Check sheet for the modelled part. Datum: model origin and axes. Units: mm. Face numbers are marked on the shaded views. A direction names the side the tool comes from. Give positions to 0.01 mm unless a question says otherwise; leave off trailing zeros. Write each loop counter-clockwise with the first axis right and the second up, starting at its lowest first coordinate (ties: lowest second). Pieces come first, ordered by that corner, then holes. Notation, with made-up numbers: (8.25, -1) -> (44.25, -1) arc R6 ccw to (44.25, 10) -> close; hole circle Ø10 at (27, 5.5). An arc over 180 degrees is marked (long way). Answer as a JSON object with one key per item and string values.
from build123d import *

# Parameters (mm, degrees)
SKETCH1_W           = 25
SKETCH1_H           = 50
SKETCH1_R           = 3.4
BOSS_EXTRUDE1_DEPTH = 3
SKETCH2_W           = 50
SKETCH2_H           = 3
BOSS_EXTRUDE2_DEPTH = 8
SKETCH3_W           = 8
SKETCH3_H           = 50
BOSS_EXTRUDE3_DEPTH = 42
SKETCH4_R           = 2.65
CUT_EXTRUDE1_DEPTH  = 0.5
SKETCH5_R           = 5.802370205
CUT_EXTRUDE2_DEPTH  = 9
FILLET2_R           = 1
SKETCH6_R           = 12.6
BOSS_EXTRUDE4_DEPTH = 2
FILLET4_R           = 1
SKETCH8_R           = 1.589780168
SKETCH8_R_2         = 1.777428262
CUT_EXTRUDE3_DEPTH  = 10
SKETCH9_W           = 49.021678163
SKETCH9_H           = 20.976854622
CUT_EXTRUDE4_DEPTH  = 68.79439129
SKETCH11_R          = 2.1
CUT_EXTRUDE5_DEPTH  = 59.480168703
SKETCH14_R          = 2.6
CUT_EXTRUDE6_DEPTH  = 0.5
CUT_EXTRUDE7_DEPTH  = 10


with BuildPart() as part:
    # Sketch1 → Boss-Extrude1 (new body)
    with BuildSketch(Plane(origin=(0, 0, 0), x_dir=(1, 0, 0), z_dir=(0, 1, 0))):
        with Locations((2.276951673, 11.384758364)):
            Rectangle(SKETCH1_W, SKETCH1_H)
        with Locations(Location((1.276951673, 11.384758364, 0), (0, 0, 270))):
            Circle(SKETCH1_R, mode=Mode.SUBTRACT)
    extrude(amount=BOSS_EXTRUDE1_DEPTH)

    # Sketch2 → Boss-Extrude2 (add)
    with BuildSketch(Plane.ZY.offset(10.223048327)):
        with Locations((-11.384758364, 1.5)):
            Rectangle(SKETCH2_W, SKETCH2_H)
    extrude(amount=BOSS_EXTRUDE2_DEPTH)

    # Sketch3 → Boss-Extrude3 (add)
    with BuildSketch(Plane.XZ):
        with Locations((-14.223048327, -11.384758364)):
            Rectangle(SKETCH3_W, SKETCH3_H)
    extrude(amount=BOSS_EXTRUDE3_DEPTH)

    # Sketch4 → Cut-Extrude1 (cut)
    with BuildSketch(Plane(origin=(0, 3, 0), x_dir=(1, 0, 0), z_dir=(0, 1, 0))):
        with Locations(Location((-14.223048327, 32.384758364, 0), (0, 0, 270))):
            Circle(SKETCH4_R)
        with Locations(Location((-14.223048327, -9.615241636, 0), (0, 0, 270))):
            Circle(SKETCH4_R)
    cut_extrude1 = extrude(amount=-CUT_EXTRUDE1_DEPTH, mode=Mode.SUBTRACT)

    # Mirror1: Cut-Extrude1 across plane
    add(cut_extrude1.mirror(Plane.ZX.offset(-19.5)), mode=Mode.SUBTRACT)

    # Sketch5 → Cut-Extrude2 (cut)
    with BuildSketch(Plane.ZY.offset(18.223048327)):
        with Locations((-11.836279124, -21)):
            Circle(SKETCH5_R)
    extrude(amount=-CUT_EXTRUDE2_DEPTH, mode=Mode.SUBTRACT)

    # Fillet2
    fillet2_edges = [part.edges().sort_by_distance(p)[0] for p in [
        (-10.223048327, -21, -17.638649329),
    ]]
    fillet(fillet2_edges, radius=FILLET2_R)

    # Mirror2: Cut-Extrude1 across plane
    add(cut_extrude1.mirror(Plane.ZY.offset(1.723048327)), mode=Mode.SUBTRACT)

    # Sketch6 → Boss-Extrude4 (add)
    with BuildSketch(Plane(origin=(0, 3, 0), x_dir=(1, 0, 0), z_dir=(0, 1, 0))):
        with BuildLine():
            Line((14.776951673, 5.825082115), (14.776951673, 16.944434614))
            ThreePointArc((14.776951673, 16.944434614), (-13.323048327, 11.384758364), (14.776951673, 5.825082115))
        make_face()
        with Locations(Location((1.276951673, 11.384758364, 0), (0, 0, 270))):
            Circle(SKETCH6_R, mode=Mode.SUBTRACT)
    extrude(amount=BOSS_EXTRUDE4_DEPTH)

    # Fillet4
    # the kernel refuses this fillet: 1 mm, written as the material it takes off along each edge
    with BuildSketch(Plane(origin=(14.776951673, 5, -3.325082115), x_dir=(0, -1, 0), z_dir=(0, 0, -1))) as fillet4_piece_1:
        with BuildLine():
            CenterArc((FILLET4_R, FILLET4_R), FILLET4_R, 180, 90)
            Line((0, FILLET4_R), (0, 0))
            Line((0, 0), (FILLET4_R, 0))
        make_face()
    extrude(amount=16.119352499, mode=Mode.SUBTRACT)

    # Sketch8 → Cut-Extrude3 (cut)
    with BuildSketch(Plane(origin=(0, 3, 0), x_dir=(1, 0, 0), z_dir=(0, 1, 0))):
        with Locations(Location((1.276951673, 19.884758364, 0), (0, 0, 270))):
            Circle(SKETCH8_R)
        with Locations(Location((1.276951673, 2.884758364, 0), (0, 0, 270))):
            Circle(SKETCH8_R_2)
    extrude(amount=-CUT_EXTRUDE3_DEPTH, mode=Mode.SUBTRACT)

    # Sketch9 → Cut-Extrude4 (cut, through all)
    with BuildSketch(Plane.XY.offset(13.615241636)):
        with Locations((-9.733887409, 10.488427311)):
            Rectangle(SKETCH9_W, SKETCH9_H)
    extrude(amount=-CUT_EXTRUDE4_DEPTH, mode=Mode.SUBTRACT)

    # Sketch11 → Cut-Extrude5 (cut, through all)
    with BuildSketch(Plane(origin=(0, 0, 0), x_dir=(1, 0, 0), z_dir=(0, 1, 0))):
        with Locations(Location((-14.223048327, 32.384758364, 0), (0, 0, 270))):
            Circle(SKETCH11_R)
    cut_extrude5 = extrude(amount=-CUT_EXTRUDE5_DEPTH, mode=Mode.SUBTRACT)

    # Mirror3: Cut-Extrude5 across plane
    add(cut_extrude5.mirror(Plane.XY.offset(-11.384758364)), mode=Mode.SUBTRACT)

    # Sketch14 → Cut-Extrude6 (cut)
    with BuildSketch(Plane(origin=(0, 0, 0), x_dir=(1, 0, 0), z_dir=(0, 1, 0))):
        with Locations(Location((-14.223048327, -9.615241636, 0), (0, 0, 270))):
            Circle(SKETCH14_R)
    cut_extrude6 = extrude(amount=-CUT_EXTRUDE6_DEPTH, mode=Mode.SUBTRACT)

    # Mirror4: Cut-Extrude6 across plane
    add(cut_extrude6.mirror(Plane.XY.offset(-11.384758364)), mode=Mode.SUBTRACT)

    # Sketch15 → Cut-Extrude7 (cut)
    with BuildSketch(Plane(origin=(-10.223048327, 0, 0), x_dir=(0, 0, -1), z_dir=(1, 0, 0))):
        with BuildLine():
            ThreePointArc((-4.015241636, -4), (-6.136561979, -4.878679656), (-7.015241636, -7))
            Line((-7.015241636, -7), (-7.015241636, -16.15570602))
            ThreePointArc((-7.015241636, -16.15570602), (-6.136561979, -18.277026364), (-4.015241636, -19.15570602))
            Line((-4.015241636, -19.15570602), (3.027273521, -19.15570602))
            ThreePointArc((3.027273521, -19.15570602), (5.435051506, -14.673525074), (9.888641359, -12.213265275))
            Line((9.888641359, -12.213265275), (9.888641359, -7))
            ThreePointArc((9.888641359, -7), (9.009961702, -4.878679656), (6.888641359, -4))
            Line((6.888641359, -4), (-4.015241636, -4))
        make_face()
        with BuildLine():
            Line((13.783916889, -7), (13.783916889, -12.213265275))
            ThreePointArc((13.783916889, -12.213265275), (18.237506742, -14.673525074), (20.645284727, -19.15570602))
            Line((20.645284727, -19.15570602), (27.687799884, -19.15570602))
            ThreePointArc((27.687799884, -19.15570602), (29.809120227, -18.277026364), (30.687799884, -16.15570602))
            Line((30.687799884, -16.15570602), (30.687799884, -7))
            ThreePointArc((30.687799884, -7), (29.809120227, -4.878679656), (27.687799884, -4))
            Line((27.687799884, -4), (16.783916889, -4))
            ThreePointArc((16.783916889, -4), (14.662596546, -4.878679656), (13.783916889, -7))
        make_face()
        with BuildLine():
            ThreePointArc((20.645284727, -22.84429398), (18.237506742, -27.326474926), (13.783916889, -29.786734725))
            Line((13.783916889, -29.786734725), (13.783916889, -38))
            Line((13.783916889, -38), (27.687799884, -38))
            ThreePointArc((27.687799884, -38), (29.809120227, -37.121320344), (30.687799884, -35))
            Line((30.687799884, -35), (30.687799884, -25.84429398))
            ThreePointArc((30.687799884, -25.84429398), (29.809120227, -23.722973636), (27.687799884, -22.84429398))
            Line((27.687799884, -22.84429398), (20.645284727, -22.84429398))
        make_face()
        with BuildLine():
            ThreePointArc((9.888641359, -29.786734725), (5.435051506, -27.326474926), (3.027273521, -22.84429398))
            Line((3.027273521, -22.84429398), (-4.015241636, -22.84429398))
            ThreePointArc((-4.015241636, -22.84429398), (-6.136561979, -23.722973636), (-7.015241636, -25.84429398))
            Line((-7.015241636, -25.84429398), (-7.015241636, -35))
            ThreePointArc((-7.015241636, -35), (-6.136561979, -37.121320344), (-4.015241636, -38))
            Line((-4.015241636, -38), (9.888641359, -38))
            Line((9.888641359, -38), (9.888641359, -29.786734725))
        make_face()
    extrude(amount=-CUT_EXTRUDE7_DEPTH, mode=Mode.SUBTRACT)


solid = part.part
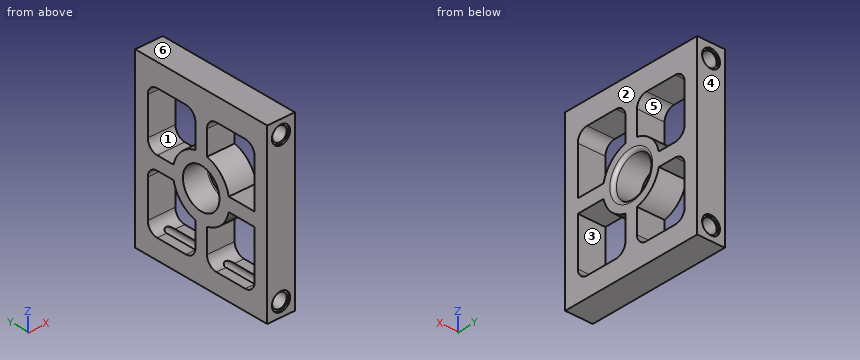
1. Mould release check, pull along Y, two halves, no side actions. Record for the marked faces 1, 2, 3 and 4: released by +Y, released by -Y, zero draft, split by the parting line, or undercut.
Determined:
{"face 1": "undercut", "face 2": "zero draft", "face 3": "undercut", "face 4": "released by +Y"}
2. Sectioned sample at D-D, the plane z = -32.5. Enter the section's corners in (x, y).
Determined:
{"outline": "(-18.22, -42) -> (-16.87, -42) -> (-16.87, -41.5) -> (-16.32, -41.5) -> (-16.32, -0.5) -> (-16.82, -0.5) -> (-16.82, 0) -> (-18.22, 0) -> close; (-12.13, -41.5) -> (-11.58, -41.5) -> (-11.58, -42) -> (-10.22, -42) -> (-10.22, 0) -> (-11.63, 0) -> (-11.63, -0.5) -> (-12.13, -0.5) -> close"}
3. Sectioned sample at B-B, the plane y = -33. Enter the section's corners in (x, z), plus the area to 3 significant figures.
Determined:
{"outline": "(-18.22, -36.38) -> (-10.22, -36.38) -> (-10.22, -30.69) -> (-12.99, -30.69) arc R2.1 cw (long way) to (-15.46, -30.69) -> (-18.22, -30.69) -> close; (-18.22, -13.78) -> (-10.22, -13.78) -> (-10.22, -9.89) -> (-18.22, -9.89) -> close; (-18.22, 7.02) -> (-10.22, 7.02) -> (-10.22, 13.62) -> (-18.22, 13.62) -> close; hole circle Ø4.2 at (-14.22, 9.62)", "area": "103 mm^2"}
4. Access from +Z, -Z, +X, -X, +Y, -Y to the whole of each face (thin tool, end or side, straight path). Record for the marked faces 5 and 6.
Determined:
{"face 5": "+X, -X", "face 6": "+Z, +X, -X, +Y, -Y"}
5. Sectioned sample at A-A, the plane z = -25. Enter the section's corners in (x, y).
Determined:
{"outline": "(-18.22, -42) -> (-10.22, -42) -> (-10.22, -38) -> (-18.22, -38) -> close; (-18.22, -22.84) -> (-10.22, -22.84) -> (-10.22, -19.16) -> (-18.22, -19.16) -> close; (-18.22, -4) -> (-10.22, -4) -> (-10.22, 0) -> (-18.22, 0) -> close"}
6. Sectioned sample at C-C, the plane y = -21. Enter the section's corners in (x, z), plus the area to 3 significant figures.
Determined:
{"outline": "(-18.22, -36.38) -> (-10.22, -36.38) -> (-10.22, -18.64) arc R1 ccw to (-11.22, -17.64) -> (-18.22, -17.64) -> close; (-18.22, -6.03) -> (-11.22, -6.03) arc R1 ccw to (-10.22, -5.03) -> (-10.22, 13.62) -> (-18.22, 13.62) -> close; hole circle Ø4.2 at (-14.22, -32.38); hole circle Ø4.2 at (-14.22, 9.62)", "area": "279 mm^2"}
7. Scan lines: L1, parallel to Y at x = -15, z = 1.5; L2, parallel to Z at x = -17.5, y = -31; L3, parallel to Z at x = -14, y = -9. Record each from-to range of solid material in increasing order. Write a range as [from, to].
Determined:
{"L1": "[-42, -38], [-22.84, -19.16], [-4, 0]", "L2": "[-36.38, -30.69], [-13.78, -9.89], [7.02, 13.62]", "L3": "[-36.38, -34.47], [-13.78, -9.89], [7.02, 7.53], [11.7, 13.62]"}
8. Go/stop test with flat-tipped pins: P1, Ø2.5, axis at x = -14, z = -32, coming from the -Y side; P2, Ø4.5, axis at x = -14.22, z = 9.62, coming from the +Y side. Record where each tip stops, or that it passes through.
Determined:
{"P1": "through", "P2": "y = -0.5"}
